Input: part model. Units: mm. Frame: model coordinates. Give positions to 0.01 mm unless a question says otherwise; leave off trailing zeros. Order: outer loops, then holes, each group sorted by start corner. A loop starts at its lowest first (then second) coordinate and runs counter-clockwise, first axis right, second up. Notation, with made-up numbers: (-19.5, 83.5) - (16.5, 83.5) arc R24 cw to (16.5, 95.5) - close; hole circle Ø1 at (63, -5). An arc over 180 degrees is marked (long way). Answer in a Markdown table with one row per item. Add a question column.
1. Section query A-A on z = 2. Return loops of the section in (x, y).
2. Section query C-C on y = -8. Return loops of the section in (x, z), and give its area (3 significant figures).
3. Contact query for flat-ended pins moving along their axis: pin 1 (2.5 mm diameter, centred on y = 12, z = 1.5, fed in from -X); pin 2 (1.4 mm diameter, centred on y = -30, z = 3, fed in from -X); pin 3 (1.4 mm diameter, centred on y = 11, z = 3.5, fed in from +X). Output: stop coordinate, or through.
4. Ray query, line 1 (X direction, y = 9.5, z = 0.2); line 2 (X direction, y = -16, z = 3.9); line 3 (X direction, y = -13.5, z = 1.2). Return the intervals inside material, ascending. Write a range as [from, to].
5. Section query B-B on x = -41. Return loops of the section in (y, z), and give its area (3 significant figures).
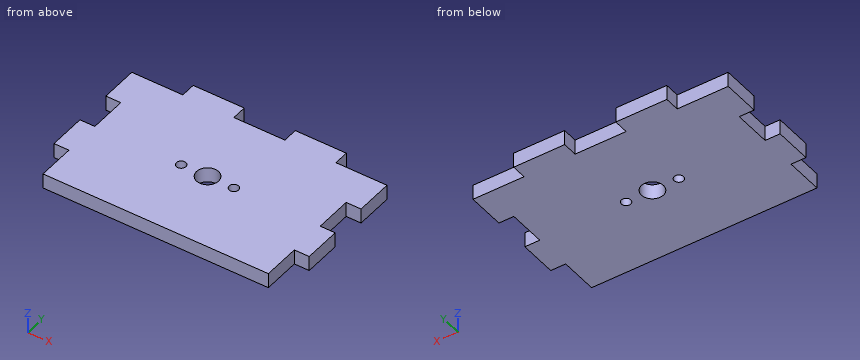
```python
from build123d import *

# Parameters (mm, degrees)
SKETCH1_W                = 82.55
SKETCH1_H                = 53.086
BOSS_EXTRUDE1_DEPTH      = 4.826
CUT_EXTRUDE1_START       = -88.085249325
CUT_EXTRUDE1_OUTLINE_W   = 4.826
CUT_EXTRUDE1_OUTLINE_H   = 4.826
CUT_EXTRUDE1_DEPTH       = 16.51
CUT_EXTRUDE1_START_2     = -55.065249325
CUT_EXTRUDE1_2_OUTLINE_W = 4.826
CUT_EXTRUDE1_2_OUTLINE_H = 4.826
CUT_EXTRUDE1_2_DEPTH     = 16.51
CUT_EXTRUDE1_START_3     = -22.045249325
CUT_EXTRUDE1_3_OUTLINE_W = 4.826
CUT_EXTRUDE1_3_OUTLINE_H = 4.826
CUT_EXTRUDE1_3_DEPTH     = 16.51
SKETCH3_W                = 4.826
SKETCH3_H                = 12.065
CUT_EXTRUDE2_DEPTH       = 97.443575108
SKETCH4_R                = 3.556
SKETCH4_R_2              = 1.524
CUT_EXTRUDE3_DEPTH       = 97.443575108


# Read off the part's stored shape, not the designer's step: Cut-Extrude1
with BuildPart() as part:
    # Sketch1 → Boss-Extrude1 (new body)
    with BuildSketch(Plane.XY):
        with Locations((-46.810249325, -12.432142782)):
            Rectangle(SKETCH1_W, SKETCH1_H)
    extrude(amount=BOSS_EXTRUDE1_DEPTH)

    # Cut-Extrude1 outline → Cut-Extrude1 (cut)
    with BuildSketch(Plane.YZ.offset(CUT_EXTRUDE1_START)):
        with Locations((11.697857218, 2.413)):
            Rectangle(CUT_EXTRUDE1_OUTLINE_W, CUT_EXTRUDE1_OUTLINE_H)
    extrude(amount=CUT_EXTRUDE1_DEPTH, mode=Mode.SUBTRACT)

    # Cut-Extrude1 2 outline → Cut-Extrude1 2 (cut)
    with BuildSketch(Plane.YZ.offset(CUT_EXTRUDE1_START_2)):
        with Locations((11.697857218, 2.413)):
            Rectangle(CUT_EXTRUDE1_2_OUTLINE_W, CUT_EXTRUDE1_2_OUTLINE_H)
    extrude(amount=CUT_EXTRUDE1_2_DEPTH, mode=Mode.SUBTRACT)

    # Cut-Extrude1 3 outline → Cut-Extrude1 3 (cut)
    with BuildSketch(Plane.YZ.offset(CUT_EXTRUDE1_START_3)):
        with Locations((11.697857218, 2.413)):
            Rectangle(CUT_EXTRUDE1_3_OUTLINE_W, CUT_EXTRUDE1_3_OUTLINE_H)
    extrude(amount=CUT_EXTRUDE1_3_DEPTH, mode=Mode.SUBTRACT)

    # Sketch3 → Cut-Extrude2 (cut, through all)
    with BuildSketch(Plane.XY.offset(4.826)):
        with Locations((-85.672249325, -32.942642782)):
            Rectangle(SKETCH3_W, SKETCH3_H)
        with Locations((-85.672249325, -8.812642782)):
            Rectangle(SKETCH3_W, SKETCH3_H)
        with Locations((-7.948249325, -32.942642782)):
            Rectangle(SKETCH3_W, SKETCH3_H)
        with Locations((-7.948249325, -8.812642782)):
            Rectangle(SKETCH3_W, SKETCH3_H)
    extrude(amount=-CUT_EXTRUDE2_DEPTH, mode=Mode.SUBTRACT)

    # Sketch4 → Cut-Extrude3 (cut, through all)
    with BuildSketch(Plane.XY.offset(4.826)):
        with Locations((-46.810249325, -14.845142782)):
            Circle(SKETCH4_R)
        with Locations((-55.331949325, -14.845142782)):
            Circle(SKETCH4_R_2)
        with Locations(Location((-38.288549325, -14.845142782, 0), (0, 0, 180))):
            Circle(SKETCH4_R_2)
    extrude(amount=-CUT_EXTRUDE3_DEPTH, mode=Mode.SUBTRACT)


solid = part.part
```
Answer:
| question | item | result |
|---|---|---|
| 1 | outline | (-88.09, -26.91) - (-83.26, -26.91) - (-83.26, -38.98) - (-10.36, -38.98) - (-10.36, -26.91) - (-5.54, -26.91) - (-5.54, -14.85) - (-10.36, -14.85) - (-10.36, -2.78) - (-5.54, -2.78) - (-5.54, 9.28) - (-22.05, 9.28) - (-22.05, 14.11) - (-38.56, 14.11) - (-38.56, 9.28) - (-55.07, 9.28) - (-55.07, 14.11) - (-71.58, 14.11) - (-71.58, 9.28) - (-88.09, 9.28) - (-88.09, -2.78) - (-83.26, -2.78) - (-83.26, -14.85) - (-88.09, -14.85) - close; hole circle Ø3.05 at (-55.33, -14.85); hole circle Ø7.11 at (-46.81, -14.85); hole circle Ø3.05 at (-38.29, -14.85) |
| 2 | outline | (-83.26, 0) - (-10.36, 0) - (-10.36, 4.83) - (-83.26, 4.83) - close |
| 2 | area | 352 mm² |
| 3 | pin 1 | stops at x = -71.58 |
| 3 | pin 2 | stops at x = -83.26 |
| 3 | pin 3 | stops at x = -22.05 |
| 4 | line 1 | x = [-71.58, -55.07], [-38.56, -22.05] |
| 4 | line 2 | x = [-88.09, -56.33], [-54.34, -50.17], [-43.45, -39.28], [-37.29, -5.54] |
| 4 | line 3 | x = [-83.26, -56.05], [-54.62, -50.1], [-43.52, -39], [-37.57, -10.36] |
| 5 | outline | (-38.98, 0) - (9.28, 0) - (9.28, 4.83) - (-38.98, 4.83) - close |
| 5 | area | 233 mm² |
